Can you work these out from the model? Positions are in its coordinate system, mm. A direction names the side the tool comes from. Give positions to 0.01 mm unless a question says otherwise; leave off trailing zeros. Write each loop counter-clockwise with the first axis right and the second up, starting at its lowest first coordinate (ties: lowest second). Pieces come first, ordered by that corner, then holes.
from build123d import *

# Parameters (mm, degrees)
F0_R     = 14.9225
F1_DEPTH = 3.4925
F2_T     = -1.5875
F3_R     = 0.254


with BuildPart() as f1:
    # F0 (on Top) → F1 (new body, symmetric)
    with BuildSketch(Plane.XY):
        Circle(F0_R)
    extrude(amount=F1_DEPTH, both=True)

    # F2
    f2_openings = [f1.faces().sort_by_distance(p)[0] for p in [
        (0, 0, 3.4925),
    ]]
    offset(amount=F2_T, openings=f2_openings)

    # F3
    f3_edges = [f1.edges().sort_by_distance(p)[0] for p in [
        (-13.335, 0, -1.905),
        (-13.335, 0, 3.4925),
        (-14.9225, 0, 3.4925),
        (-14.9225, 0, -3.4925),
    ]]
    fillet(f3_edges, radius=F3_R)


solid = f1.part
(1) Imagine slicing it at C-C, the plane z = -2.5. Write out the boundary of the cut face in (x, y) (1 decimal), plus the area to 3 significant figures.
Returned:
outline: circle Ø29.8 at (0, 0)
area: 700 mm2
(2) If we mould it in two halves opening along Y, with no side actions, what happens to faces 3 (the face through (14.233, 4.482, 0.045)), 4 (the face through (10, -10, 3.492)), 5 (the face through (-9.83, 9.01, 0.83))? For each: +Y half, -Y half, draft (parallel to the pull), parting line (faces both ways), or undercut.
Returned:
face 3: parting line
face 4: draft
face 5: undercut
(3) Will these pins go through, and if not, where does the flat tip stop? P1, Ø1, axis at x = 8, z = -2, coming from the +Y side; P2, Ø2, axis at y = -3, z = -1.5, coming from the +X side; P3, Ø4, axis at y = -3, z = 1.5, coming from the -X side.
Returned:
P1: stops at y = 12.9
P2: stops at x = 14.79
P3: stops at x = -14.89
(4) For faces 1 (the face through (0, 0, -1.905)), 2 (the face through (0, 0, -3.492)), which set-ups out of +Z, -Z, +X, -X, +Y, -Y let a thin tool reach every point of the face, with its end or its side?
Returned:
face 1: +Z
face 2: -Z, +X, -X, +Y, -Y
(5) If I drill on L1, parallel to Y at x = 0, z = -0.15 (1 decimal); L2, parallel to Y at x = -7.75, z = 0; L3, parallel to Z at x = 4.25, y = 10.5 (1 decimal), over which ranges is the centre line in solid material (lowest first)?
Returned:
L1: y = -14.9 to -13.3, 13.3 to 14.9
L2: y = -12.75 to -10.85, 10.85 to 12.75
L3: z = -3.5 to -1.9
